from build123d import *

# Parameters (mm, degrees)
BOSS_EXTRUDE1_DEPTH                             = 22.5
FILLET1_R                                       = 1
CSK_FOR_M2_FLAT_HEAD_MACHINE_SCREW1_D           = 2.4
CSK_FOR_M2_FLAT_HEAD_MACHINE_SCREW1_DEPTH       = 6.45
CSK_FOR_M2_FLAT_HEAD_MACHINE_SCREW1_CSINK_D     = 4.4
CSK_FOR_M2_FLAT_HEAD_MACHINE_SCREW1_CSINK_ANGLE = 90
CSK_FOR_M2_FLAT_HEAD_MACHINE_SCREW1_TIP         = 0.721032743
FILLET2_R                                       = 2
TAPPED_HOLE_FOR_M2_5X0_45_HELICOIL1_D           = 2.55
TAPPED_HOLE_FOR_M2_5X0_45_HELICOIL1_DEPTH       = 4
TAPPED_HOLE_FOR_M2_5X0_45_HELICOIL1_CSINK_D     = 3.195
TAPPED_HOLE_FOR_M2_5X0_45_HELICOIL1_CSINK_ANGLE = 90
TAPPED_HOLE_FOR_M2_5X0_45_HELICOIL1_TIP         = 0.766097289


with BuildPart() as part:
    # Sketch1 → Boss-Extrude1 (new, symmetric)
    with BuildSketch(Plane(origin=(0, 0, 0), x_dir=(0, 0, -1), z_dir=(1, 0, 0))):
        Polygon((0, 0), (0, 18.94), (-5, 18.94), (-5, 13.94), (-2, 13.94), (-2, 10.54), (-14.9, 10.54), (-14.9, 9.04), (-2, 9.04), (-2, 0), align=None)
    extrude(amount=BOSS_EXTRUDE1_DEPTH, both=True)

    # Fillet1
    fillet1_edges = [part.edges().sort_by_distance(p)[0] for p in [
        (0, 9.04, 2),
        (0, 10.54, 2),
        (0, 13.94, 2),
    ]]
    fillet(fillet1_edges, radius=FILLET1_R)

    # CSK for M2 Flat Head Machine Screw1
    with Locations(Plane.XY.offset(2)):
        with Locations((20, 2.3), (-20, 2.3), (0, 2.3)):
            CounterSinkHole(CSK_FOR_M2_FLAT_HEAD_MACHINE_SCREW1_D / 2, CSK_FOR_M2_FLAT_HEAD_MACHINE_SCREW1_CSINK_D / 2, depth=CSK_FOR_M2_FLAT_HEAD_MACHINE_SCREW1_DEPTH, counter_sink_angle=CSK_FOR_M2_FLAT_HEAD_MACHINE_SCREW1_CSINK_ANGLE)
            with Locations((0, 0, -(CSK_FOR_M2_FLAT_HEAD_MACHINE_SCREW1_DEPTH + CSK_FOR_M2_FLAT_HEAD_MACHINE_SCREW1_TIP / 2))):  # 118° drill point
                Cone(0, CSK_FOR_M2_FLAT_HEAD_MACHINE_SCREW1_D / 2, CSK_FOR_M2_FLAT_HEAD_MACHINE_SCREW1_TIP, mode=Mode.SUBTRACT)

    # Fillet2
    fillet2_edges = [part.edges().sort_by_distance(p)[0] for p in [
        (-22.5, 0, 1),
        (22.5, 0, 1),
    ]]
    fillet(fillet2_edges, radius=FILLET2_R)

    # Tapped Hole for M2.5x0.45 Helicoil1
    with Locations(Plane(origin=(0, 18.94, 0), x_dir=(1, 0, 0), z_dir=(0, 1, 0))):
        with Locations((20, -2.5), (-20, -2.5), (0, -2.5)):
            CounterSinkHole(TAPPED_HOLE_FOR_M2_5X0_45_HELICOIL1_D / 2, TAPPED_HOLE_FOR_M2_5X0_45_HELICOIL1_CSINK_D / 2, depth=TAPPED_HOLE_FOR_M2_5X0_45_HELICOIL1_DEPTH, counter_sink_angle=TAPPED_HOLE_FOR_M2_5X0_45_HELICOIL1_CSINK_ANGLE)
            with Locations((0, 0, -(TAPPED_HOLE_FOR_M2_5X0_45_HELICOIL1_DEPTH + TAPPED_HOLE_FOR_M2_5X0_45_HELICOIL1_TIP / 2))):  # 118° drill point
                Cone(0, TAPPED_HOLE_FOR_M2_5X0_45_HELICOIL1_D / 2, TAPPED_HOLE_FOR_M2_5X0_45_HELICOIL1_TIP, mode=Mode.SUBTRACT)


solid = part.part
Geometry check sheet. Reference: the model listing, model coordinates, mm. A direction names the side the tool comes from. Round coordinates to 2 decimals unless told otherwise and drop trailing zeros. Order: outer loops, then holes, each group sorted by start corner. A loop starts at its lowest first (then second) coordinate and runs counter-clockwise, first axis right, second up. Notation, with made-up numbers: M 7,-34.75 L 12,-34.75 A29 cw 12,-1.75 Z; hole C 33,37.25 d9. An arc over 180 degrees is marked long. Answer in a Markdown table with one row per item. Add a question column.
Item 1: Sectioned sample at C-C, the plane z = 13. Enter the section's corners in (x, y), plus the area to 3 significant figures.
Item 2: Depth check by flat-ended pin: pin 1 Ø3 at (y, z) = (11.5, 2.5) entering from -X; pin 2 Ø1.6 at (x, z) = (7, 4) entering from -Y; pin 3 Ø6.5 at (x, y) = (-0.5, 3) entering from +Z; pin 4 Ø1.9 at (x, y) = (0, 2.3) entering from -Z. Enter the tip coordinate at first touch or a pass-through.
Item 3: Draft check along X on faces 1 (the face through (0, 0, 1)), 2 (the face through (-18.726, 16.753, 2.444)), 3 (the face through (-21.9, 0.57, 0.99)), 4 (the face through (-0.685, 16.753, 1.425)). Enter one of: released by +X, released by -X, zero draft, split by the parting line, or undercut.
Item 4: Material ranges on L1, parallel to X at y = 2.3, z = 0.35; L2, parallel to Z at x = 0, y = 16.6 (3 decimals); L3, parallel to Y at x = 20, z = 0.5, recorded low to high. Write a range as [from, to].
Item 5: Sectioned sample at B-B, the plane x = 7.5. Enter the section's corners in (y, z), plus the area to 3 significant figures.
Item 6: Set-up check for faces 5 (the face through (0, 16, 5)), 6 (the face through (0.315, 10.825, 2.301)), 7 (the face through (21.274, 16.753, 2.444)): record each of +Z, -Z, +X, -X, +Y, -Y from which the full face is reachable in a straight line by a thin tool's end or side.
Item 7: Sectioned sample at A-A, the plane y = 15.5. Enter the section's corners in (x, z) (3 decimals), plus the area to 3 significant figures.
Filled in:
| question | item | result |
|---|---|---|
| 1 | outline | M -22.5,9.04 L 22.5,9.04 L 22.5,10.54 L -22.5,10.54 Z |
| 1 | area | 67.5 mm² |
| 2 | pin 1 | stops at x = -22.5 |
| 2 | pin 2 | stops at y = 9.04 |
| 2 | pin 3 | stops at z = 2 |
| 2 | pin 4 | passes through |
| 3 | face 1 | zero draft |
| 3 | face 2 | undercut |
| 3 | face 3 | released by -X |
| 3 | face 4 | undercut |
| 4 | L1 | x = [-22.5, -21.2], [-18.8, -1.2], [1.2, 18.8], [21.2, 22.5] |
| 4 | L2 | z = [0, 1.225], [3.775, 5] |
| 4 | L3 | y = [0, 1.1], [3.5, 18.94] |
| 5 | outline | M 0,0 L 18.94,0 L 18.94,5 L 13.94,5 L 13.94,3 A1 cw 12.94,2 L 11.54,2 A1 cw 10.54,3 L 10.54,14.9 L 9.04,14.9 L 9.04,3 A1 cw 8.04,2 L 0,2 Z |
| 5 | area | 72.9 mm² |
| 6 | face 5 | +Z, +X, -X, +Y |
| 6 | face 6 | +Z, +X, -X |
| 6 | face 7 | +Y |
| 7 | outline | M -22.5,0 L 22.5,0 L 22.5,5 L -22.5,5 Z; hole C -20,2.5 d2.55; hole C 0,2.5 d2.55; hole C 20,2.5 d2.55 |
| 7 | area | 210 mm² |
